Check sheet for the drawn part. Datum: minimum x, y, z corner. Units: mm. A direction names the side the tool comes from. Coordinates: 2 decimals unless noted, no trailing zeros. Write each loop counter-clockwise with the first axis right and the second up, starting at its lowest first coordinate (ties: lowest second). Pieces come first, ordered by that corner, then holes. Notation, with made-up numbers: (87.25, -3) -> (135.25, -3) arc R34 ccw to (135.25, 32) -> close; hole circle Ø2 at (-31.5, -12). An arc over 180 degrees is marked (long way). Write item = value, one per line. Start each with the question number.
(1) Section check B-B (y = 2.4). Record the cut outline in (x, z).
(2) Set-up check for the marked faces 1, 2 and 3: record each of +Z, -Z, +X, -X, +Y, -Y from which the full face is reachable in a straight line by a thin tool's end or side.
(3) Section check A-A (z = 2.8). Record the cut outline in (x, y), plus the area to 3 significant figures.
(4) Section check C-C (y = 3.35). Record the cut outline in (x, z).
(5) Material ranges on probe 1 along Y at (x, z) = (1.5, 2.05); probe 2 along X at (y, z) = (0.75, 2.7); probe 3 along Y at (x, z) = (14, 1.3), recorded low to high. Write a range as [from, to].
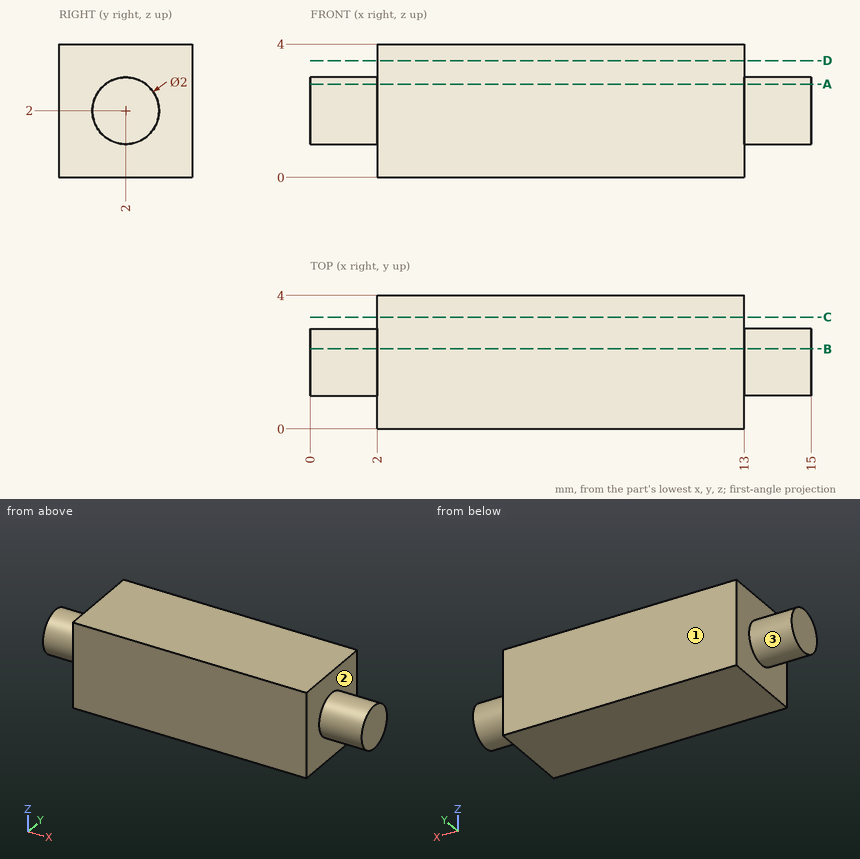
Response:
q1.outline = (0, 1.08) -> (2, 1.08) -> (2, 0) -> (13, 0) -> (13, 1.08) -> (15, 1.08) -> (15, 2.92) -> (13, 2.92) -> (13, 4) -> (2, 4) -> (2, 2.92) -> (0, 2.92) -> close
q2.face_1 = +Z, -Z, +X, -X, +Y
q2.face_2 = +X
q2.face_3 = -X
q3.outline = (0, 1.4) -> (2, 1.4) -> (2, 0) -> (13, 0) -> (13, 1.4) -> (15, 1.4) -> (15, 2.6) -> (13, 2.6) -> (13, 4) -> (2, 4) -> (2, 2.6) -> (0, 2.6) -> close
q3.area = 48.8 mm2
q4.outline = (2, 0) -> (13, 0) -> (13, 4) -> (2, 4) -> close
q5.probe_1 = [1, 3]
q5.probe_2 = [2, 13]
q5.probe_3 = [1.29, 2.71]
